Can you work these out from the model? Positions are in its coordinate system, mm. A direction names the side the tool comes from. Coordinates: 2 decimals unless noted, no trailing zeros. Loops run counter-clockwise (first coordinate to the right, second up) from the corner with the lowest first, then second, coordinate; pieces in that order, holes last.
Autodesk Inventor part; units mm, degrees
ref_plane "YZ Plane" through (0, 0, 0) normal (1, 0, 0) x (0, 1, 0)
ref_plane "XZ Plane" through (0, 0, 0) normal (0, 1, 0) x (-1, 0, 0)
ref_plane "XY Plane" through (0, 0, 0) normal (0, 0, 1) x (1, 0, 0)
sketch "Sketch1" plane through (0, 0, 0) normal (0, 1, 0) x (-1, 0, 0)
  circle A0 centre (0, 0) radius 1.675
  dimension "d0" = 3.35
extrude "Extrusion1" add sketch "Sketch1" along normal blind 8
sketch "Sketch2" plane through (0, 8, 0) normal (0, 1, 0) x (1, 0, 0)
  circle A0 centre (0, 0) radius 1.675
  circle A1 centre (0, 0) radius 2.925
  dimension "d3" = 5.85
extrude "Extrusion2" add sketch "Sketch2" along normal blind 3 contours A0 | A1
sketch "Sketch3" plane through (0, 11, 0) normal (0, 1, 0) x (1, 0, 0)
  line L0 (-0.8268, 1.1831) -> (0.6112, 1.3076)
  line L1 (0.6112, 1.3076) -> (1.438, 0.1244)
  line L2 (1.438, 0.1244) -> (0.8268, -1.1831)
  line L3 (0.8268, -1.1831) -> (-0.6112, -1.3076)
  line L4 (-0.6112, -1.3076) -> (-1.438, -0.1244)
  line L5 (-1.438, -0.1244) -> (-0.8268, 1.1831)
  point P0 (0, 0)
  point P1 (0, 0)
  dimension "d6" = 2.5
extrude "Extrusion3" cut sketch "Sketch3" against normal blind 1.9
equation "\"d0\" = screw_m3_A"
equation "\"d1\" = screw_m3_B"
equation "\"d3\" = screw_m3_C"
equation "\"d4\" = screw_m3_D"
equation "\"screw_m3_B\" = 8"
equation "\"screw_m3_D\" = 3"
properties part number "M3_SCREW_8MM"
(1) If I drill on probe 1 along Y at (x, z) = (-0.85, -0.3); probe 2 along Y at (x, z) = (-1.35, -2.3); probe 3 along X at (y, z) = (9, 0.45), over which ranges is the centre line in solid material (lowest first)?
Check values:
probe 1: y = 0 to 9.1
probe 2: y = 8 to 11
probe 3: x = -2.89 to 2.89
(2) I want a section at B-B on x = 0. Write out the boundary of the cut face in (y, z) (3 decimals).
Check values:
outline: (0, -1.675) - (8, -1.675) - (8, -2.925) - (11, -2.925) - (11, -1.255) - (9.1, -1.255) - (9.1, 1.255) - (11, 1.255) - (11, 2.925) - (8, 2.925) - (8, 1.675) - (0, 1.675) - close
(3) If we mould it in two halves opening along Z, with no side actions, what happens to faces 4 (the cylindrical face through (-0.634, 9.479, -2.855)), 5 (the flat face through (0, 0, 0)), 6 (the flat face through (0.118, 10.063, 1.244))? For each: released by +Z, released by -Z, zero draft, split by the parting line, or undercut.
Check values:
face 4: split by the parting line
face 5: zero draft
face 6: undercut
(4) I want a section at D-D on x = 2.2. Write out the boundary of the cut face in (y, z).
Check values:
outline: (8, -1.93) - (11, -1.93) - (11, 1.93) - (8, 1.93) - close
(5) I'm going to push flat-ended pins straight in: pin 1 (1 mm diameter, centred on y = 4.5, z = 0.5, fed in from +X) (3 decimals); pin 2 (1.5 mm diameter, centred on y = 1.5, z = 2, fed in from -X); pin 3 (3 mm diameter, centred on x = 0.5, z = 0, fed in from +Y); pin 4 (1 mm diameter, centred on x = 1, y = 3.5, fed in from -Z). Where does each tip first touch, or does it pass through?
Check values:
pin 1: stops at x = 1.675
pin 2: stops at x = -1.11
pin 3: stops at y = 11
pin 4: stops at z = -1.6
(6) I want a section at C-C on y = 2.5. Write out the boundary of the cut face in (x, z) (3 decimals), then the cut area to 3 significant figures.
Check values:
outline: circle Ø3.35 at (0, 0)
area: 8.81 mm2
(7) I want a section at A-A on z = 0. Write out the boundary of the cut face in (x, y) (3 decimals).
Check values:
outline: (-2.925, 8) - (-1.675, 8) - (-1.675, 0) - (1.675, 0) - (1.675, 8) - (2.925, 8) - (2.925, 11) - (1.38, 11) - (1.38, 9.1) - (-1.38, 9.1) - (-1.38, 11) - (-2.925, 11) - close
(8) Which directions (+Z, -Z, +X, -X, +Y, -Y) give clear straight access to the entire face, cutting with the end or side of a thin tool? Please do faces 1 (the cylindrical face through (1.673, 3.944, -0.074)), 2 (the flat face through (1.3, 11, 0.6)), 3 (the flat face through (-1.137, 10.063, -0.52)).
Check values:
face 1: -Y
face 2: +Z, -Z, +X, -X, +Y
face 3: +Y
